Could you check a few things on this model? Use its own coordinates, in mm. Face numbers are marked on the shaded views. A direction names the side the tool comes from. Coordinates: 2 decimals unless noted, no trailing zeros. Order: outer loops, then holes, each group sorted by start corner. A loop starts at its lowest first (then second) coordinate and runs counter-clockwise, first axis right, second up.
```python
from build123d import *

# Parameters (mm, degrees)
SKETCH1_W           = 45
SKETCH1_H           = 20
BOSS_EXTRUDE1_DEPTH = 1.5
SKETCH2_R           = 3
BOSS_EXTRUDE3_DEPTH = 8
SKETCH3_W           = 10
SKETCH3_H           = 3
BOSS_EXTRUDE4_DEPTH = 9
BOSS_EXTRUDE5_DEPTH = 6
SKETCH6_W           = 9
SKETCH6_H           = 7.5
BOSS_EXTRUDE6_DEPTH = 2.5
SKETCH7_W           = 3
SKETCH7_H           = 1.5
BOSS_EXTRUDE7_DEPTH = 1.5
SKETCH9_R           = 1.25
CUT_EXTRUDE1_DEPTH  = 27.215453458
SKETCH10_R          = 1.25
CUT_EXTRUDE2_DEPTH  = 27.215453458
SKETCH12_R          = 0.25
CUT_EXTRUDE3_DEPTH  = 1.5


with BuildPart() as part:
    # Sketch1 → Boss-Extrude1 (new body)
    with BuildSketch(Plane.XY):
        Rectangle(SKETCH1_W, SKETCH1_H)
    extrude(amount=BOSS_EXTRUDE1_DEPTH)

    # Sketch2 → Boss-Extrude3 (add)
    with BuildSketch(Plane.XY.offset(1.5)):
        with Locations((-18.5, 0)):
            Circle(SKETCH2_R)
        with Locations(Location((18.5, 0, 0), (0, 0, 180))):
            Circle(SKETCH2_R)
    extrude(amount=BOSS_EXTRUDE3_DEPTH)

    # Sketch3 → Boss-Extrude4 (add)
    with BuildSketch(Plane.XY.offset(1.5)):
        with Locations((-8.5, 6)):
            Rectangle(SKETCH3_W, SKETCH3_H)
    extrude(amount=BOSS_EXTRUDE4_DEPTH)

    # Sketch5 → Boss-Extrude5 (add)
    with BuildSketch(Plane.XY.offset(1.5)):
        with BuildLine():
            Line((-12, 1), (-4, 1))
            ThreePointArc((-4, 1), (-2.585786438, 0.414213562), (-2, -1))
            Line((-2, -1), (-2, -6))
            ThreePointArc((-2, -6), (-2.585786438, -7.414213562), (-4, -8))
            Line((-4, -8), (-12, -8))
            ThreePointArc((-12, -8), (-13.414213562, -7.414213562), (-14, -6))
            Line((-14, -6), (-14, -1))
            ThreePointArc((-14, -1), (-13.414213562, 0.414213562), (-12, 1))
        make_face()
    extrude(amount=BOSS_EXTRUDE5_DEPTH)

    # Sketch6 → Boss-Extrude6 (add)
    with BuildSketch(Plane.XY.offset(1.5)):
        with Locations((7, 3.75)):
            Rectangle(SKETCH6_W, SKETCH6_H)
    extrude(amount=BOSS_EXTRUDE6_DEPTH)

    # Sketch7 → Boss-Extrude7 (add)
    with BuildSketch(Plane.XY.offset(1.5)):
        with Locations((10, -5.25)):
            Rectangle(SKETCH7_W, SKETCH7_H)
    extrude(amount=BOSS_EXTRUDE7_DEPTH)

    # Sketch9 → Cut-Extrude1 (cut, through all)
    with BuildSketch(Plane.XY.offset(1.5)):
        with Locations((-17.5, -7)):
            Circle(SKETCH9_R)
        with Locations(Location((-17.5, 7, 0), (0, 0, 180))):
            Circle(SKETCH9_R)
    extrude(amount=-CUT_EXTRUDE1_DEPTH, mode=Mode.SUBTRACT)

    # Sketch10 → Cut-Extrude2 (cut, through all)
    with BuildSketch(Plane.XY.offset(1.5)):
        with Locations((16, 6.5)):
            Circle(SKETCH10_R)
        with Locations(Location((16, -6.5, 0), (0, 0, 180))):
            Circle(SKETCH10_R)
    extrude(amount=-CUT_EXTRUDE2_DEPTH, mode=Mode.SUBTRACT)

    # Sketch12 → Cut-Extrude3 (cut)
    with BuildSketch(Plane.XY.offset(1.5)):
        with Locations((-21.5, 9)):
            Circle(SKETCH12_R)
        with Locations((21.5, 9)):
            Circle(SKETCH12_R)
        with Locations((21.5, -9)):
            Circle(SKETCH12_R)
        with Locations((-21.5, -9)):
            Circle(SKETCH12_R)
    extrude(amount=-CUT_EXTRUDE3_DEPTH, mode=Mode.SUBTRACT)


solid = part.part
```
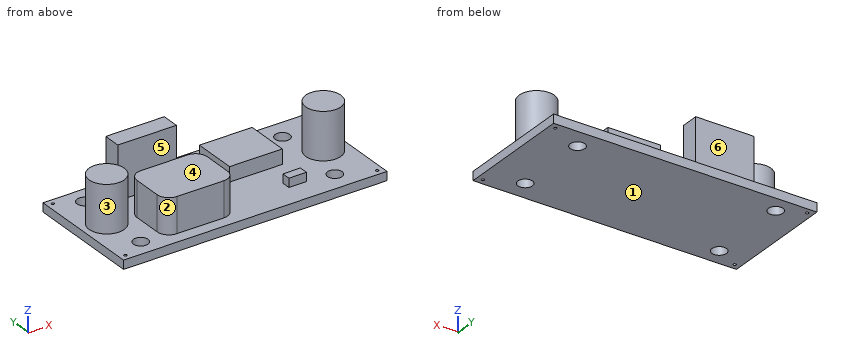
Item 1: I need wall thicknesses on line 1 (Y direction, x = 21.5, z = 0.65); line 2 (Y direction, x = -17.5, z = 0.95); line 3 (X direction, y = 7, z = 1.1). Which ranges of each line are inside material? Lowest first, please.
Item 2: Suppose I cut it at C-C (z = 2.5). List the corners of the cut face in (x, y) for me.
Item 3: Suppose I cut it at A-A (z = 6.75). List the corners of the cut face in (x, y) for me.
Item 4: Suppose I cut it at B-B (y = 6.5). List the corners of the cut face in (x, z) for me, and give its area (3 significant figures).
Item 5: Thinking about a two-plate mould opening in X: for the marked faces 1, 2 and 3, which applies, +X half, -X half, draft (parallel to the pull), parting line (faces both ways), or undercut?
Item 6: Suppose I cut it at D-D (x = -17.5). List the corners of the cut face in (y, z) for me.
Item 7: Which directions (+Z, -Z, +X, -X, +Y, -Y) give clear straight access to the entire face, cutting with the end or side of a thin tool? Please do the marked faces 4, 5 and 6.
Item 8: For pin 1 Ø4 at (x, z) = (3.5, 6.5) entering from -Y; pin 2 Ø3 at (x, y) = (-17.5, 7) entering from -Z; pin 3 Ø7 at (x, y) = (-9.5, -3.5) entering from +Z; pin 4 Ø0.8 at (y, z) = (4, 3) entering from -X, each with a flat end and sliding along its axis, tell me the tip position at first contact or that it passes through.
Geometry results:
1. line 1: y = -10 to -9.25, -8.75 to 8.75, 9.25 to 10
1. line 2: y = -10 to -8.25, -5.75 to 5.75, 8.25 to 10
1. line 3: x = -22.5 to -18.75, -16.25 to 14.85, 17.15 to 22.5
2. outline: circle Ø6 at (-18.5, 0); (-14, -6) arc R2 ccw to (-12, -8) - (-4, -8) arc R2 ccw to (-2, -6) - (-2, -1) arc R2 ccw to (-4, 1) - (-12, 1) arc R2 ccw to (-14, -1) - close; (-13.5, 4.5) - (-3.5, 4.5) - (-3.5, 7.5) - (-13.5, 7.5) - close; (2.5, 0) - (11.5, 0) - (11.5, 7.5) - (2.5, 7.5) - close; (8.5, -6) - (11.5, -6) - (11.5, -4.5) - (8.5, -4.5) - close; circle Ø6 at (18.5, 0)
3. outline: circle Ø6 at (-18.5, 0); (-14, -6) arc R2 ccw to (-12, -8) - (-4, -8) arc R2 ccw to (-2, -6) - (-2, -1) arc R2 ccw to (-4, 1) - (-12, 1) arc R2 ccw to (-14, -1) - close; (-13.5, 4.5) - (-3.5, 4.5) - (-3.5, 7.5) - (-13.5, 7.5) - close; circle Ø6 at (18.5, 0)
4. outline: (-22.5, 0) - (-18.65, 0) - (-18.65, 1.5) - (-22.5, 1.5) - close; (-16.35, 0) - (14.75, 0) - (14.75, 1.5) - (11.5, 1.5) - (11.5, 4) - (2.5, 4) - (2.5, 1.5) - (-3.5, 1.5) - (-3.5, 10.5) - (-13.5, 10.5) - (-13.5, 1.5) - (-16.35, 1.5) - close; (17.25, 0) - (22.5, 0) - (22.5, 1.5) - (17.25, 1.5) - close
4. area: 173 mm2
5. face 1: draft
5. face 2: -X half
5. face 3: undercut
6. outline: (-10, 0) - (-8.25, 0) - (-8.25, 1.5) - (-10, 1.5) - close; (-5.75, 0) - (5.75, 0) - (5.75, 1.5) - (2.83, 1.5) - (2.83, 9.5) - (-2.83, 9.5) - (-2.83, 1.5) - (-5.75, 1.5) - close; (8.25, 0) - (10, 0) - (10, 1.5) - (8.25, 1.5) - close
7. face 4: +Z, -Y
7. face 5: +Z, -X
7. face 6: +Z, +X, -X, +Y
8. pin 1: passes through
8. pin 2: stops at z = 0
8. pin 3: stops at z = 7.5
8. pin 4: stops at x = 2.5
